from build123d import *

# Parameters (mm, degrees)
F0_W     = 42.9938789457
F0_H     = 54.2596541345
F1_DEPTH = 25.4
F3_D     = 6.35
F6_SIZE  = 5.08


# Not quite as in the source:
# - the program builds the solid bodies; features that only make, move or delete a surface that nothing else refers to are left out


with BuildPart() as f1:
    # F0 (on Front) → F1 (new body)
    with BuildSketch(Plane.XZ):
        with Locations((8.1619387493, -0.9196549654)):
            Rectangle(F0_W, F0_H)
    extrude(amount=F1_DEPTH)

    # F3 (through all)
    with Locations(Plane.XZ.offset(25.4)):
        with Locations((7.9346429557, 12.5517835841)):
            Hole(F3_D / 2)

    # F6
    f6_edges = [f1.edges().sort_by_distance(p)[0] for p in [
        (8.161939, -25.4, 26.210172),
    ]]
    chamfer(f6_edges, length=F6_SIZE)


solid = f1.part
The listing builds one solid part. Answer for the finished solid, in the listing's coordinates (mm). Coordinates: 2 decimals unless noted, no trailing zeros. Loops run counter-clockwise (first coordinate to the right, second up) from the corner with the lowest first, then second, coordinate; pieces in that order, holes last. Notation, with made-up numbers: M -27,69 L 20,69 A19 ccw 20,90 Z; hole C 62,52 d10. An arc over 180 degrees is marked long. Answer in a Markdown table with one row per item.
1) Given pin 1 (10 mm diameter, centred on x = 7.93, z = 12.55, fed in from +Y), flat-ended and moving along its own axis, determine where the tip first touches the part or whether it passes through.
Answers below:
| item | result |
|---|---|
| pin 1 | y = 0 |
2) Find section B-B (z = 23). Determine the outline of the cut face in (x, y) (3 decimals).
Answers below:
| item | result |
|---|---|
| outline | M -13.335,-23.53 L 29.659,-23.53 L 29.659,0 L -13.335,0 Z |
3) Find the intervals of material crossed by probe 1 along X at (y, z) = (-20.75, 11) (3 decimals); probe 2 along Z at (x, y) = (9.5, -4.5), in increasing order.
Answers below:
| item | result |
|---|---|
| probe 1 | -13.335 to 5.165, 10.705 to 29.659 |
| probe 2 | -28.05 to 9.79, 15.31 to 26.21 |
4) Determine the mould class of faces 1 (the flat face through (8, -10, 26.21)), 2 (the cylindrical face through (6.47, -12.522, 9.735)), 3 (the flat face through (8, -13, -28.049)) for opening direction Z: released by +Z, released by -Z, zero draft, split by the parting line, or undercut.
Answers below:
| item | result |
|---|---|
| face 1 | released by +Z |
| face 2 | undercut |
| face 3 | released by -Z |
5) Find section A-A (z = 11). Determine the outline of the cut face in (x, y) (3 decimals), then the cut area to 3 significant figures.
Answers below:
| item | result |
|---|---|
| outline | M -13.335,-25.4 L 5.165,-25.4 L 5.165,0 L -13.335,0 Z; M 10.705,-25.4 L 29.659,-25.4 L 29.659,0 L 10.705,0 Z |
| area | 951 mm^2 |
